from build123d import *

# Parameters (mm, degrees)
BOSS_EXTRUDE1_DEPTH = 8
SKETCH2_R           = 4.5
BOSS_EXTRUDE2_DEPTH = 7
CUT_EXTRUDE1_DEPTH  = 5.5
FILLET1_R           = 0.5
CHAMFER1_SIZE       = 0.25


with BuildPart() as part:
    # Sketch1 → Boss-Extrude1 (new body)
    with BuildSketch(Plane(origin=(0, 0, 0), x_dir=(1, 0, 0), z_dir=(0, 1, 0))):
        with BuildLine():
            Line((-1.75, 2.056088519), (-1.75, -2.056088519))
            ThreePointArc((-1.75, -2.056088519), (0, -2.7), (1.75, -2.056088519))
            Line((1.75, -2.056088519), (1.75, 2.056088519))
            ThreePointArc((1.75, 2.056088519), (0, 2.7), (-1.75, 2.056088519))
        make_face()
    extrude(amount=BOSS_EXTRUDE1_DEPTH)

    # Sketch2 → Boss-Extrude2 (add)
    with BuildSketch(Plane(origin=(0, 8, 0), x_dir=(1, 0, 0), z_dir=(0, 1, 0))):
        Circle(SKETCH2_R)
    extrude(amount=BOSS_EXTRUDE2_DEPTH)

    # Sketch3 → Cut-Extrude1 (cut)
    with BuildSketch(Plane(origin=(0, 15, 0), x_dir=(1, 0, 0), z_dir=(0, 1, 0))):
        with BuildLine():
            Line((-1.322875656, 1.5), (1.322875656, 1.5))
            ThreePointArc((1.322875656, 1.5), (0, -2), (-1.322875656, 1.5))
        make_face()
    extrude(amount=-CUT_EXTRUDE1_DEPTH, mode=Mode.SUBTRACT)

    # Fillet1
    fillet1_edges = [part.edges().sort_by_distance(p)[0] for p in [
        (0, 8, 2.7),
        (1.75, 8, 0),
        (0, 8, -2.7),
        (-1.75, 8, 0),
    ]]
    fillet(fillet1_edges, radius=FILLET1_R)

    # Chamfer1
    chamfer1_edges = [part.edges().sort_by_distance(p)[0] for p in [
        (-4.5, 8, 0),
        (-4.5, 15, 0),
        (0, 15, 2),
        (0, 15, -1.5),
        (1.75, 0, 0),
        (0, 0, 2.7),
        (-1.75, 0, 0),
        (0, 0, -2.7),
    ]]
    chamfer(chamfer1_edges, length=CHAMFER1_SIZE)


solid = part.part
Work out the finished part from the listing and answer in its coordinate system (mm). A direction names the side the tool comes from. Give positions to 0.01 mm unless a question says otherwise; leave off trailing zeros. Loops run counter-clockwise (first coordinate to the right, second up) from the corner with the lowest first, then second, coordinate; pieces in that order, holes last. Notation, with made-up numbers: (47, 56) -> (73, 56) arc R22 cw to (73, 64) -> close; hole circle Ø10 at (75.25, 89.5). An arc over 180 degrees is marked (long way). Use a Markdown table: item, result. Add a question column.
1. Section C-C on y = 5 is taken. Determine the outline of the cut face in (x, z), and give its area (3 significant figures).
2. Find the intervals of material crossed by probe 1 along X at (y, z) = (10.85, 0); probe 2 along Y at (x, z) = (0.25, 0); probe 3 along Y at (x, z) = (-3, 2), in increasing order.
3. Flat-ended cylindrical pins translate along their axes: pin 1 Ø4 at (x, y) = (-0.5, 11.5) entering from +Z; pin 2 Ø1.2 at (y, z) = (5.5, 0.5) entering from +X; pin 3 Ø1.2 at (y, z) = (3, -0.5) entering from -X; pin 4 Ø1.5 at (x, y) = (-1.5, 3.5) entering from +Z. Find the tip coordinate at first contact, or state that the pin passes through.
4. Section A-A on x = 0 is taken. Determine the outline of the cut face in (y, z), and give its area (3 significant figures).
5. Section B-B on z = 0 is taken. Determine the outline of the cut face in (x, y).
6. Determine the mould class of faces 1 (the cylindrical face through (0, 3.8, 2.7)), 2 (the flat face through (-1.75, 4, 0)), 3 (the cylindrical face through (0, 12, 2)) for opening direction Z: released by +Z, released by -Z, zero draft, split by the parting line, or undercut.
7. For faces 4 (the flat face through (3, 8, 0)), 5 (the flat face through (1.75, 4, 0)), 6 (the cylindrical face through (0, 3.8, -2.7)), 7 (the flat face through (0, 12, -1.5)), determine the directions among +Z, -Z, +X, -X, +Y, -Y from which every point of the face is accessible in a straight line to the end or side of a thin tool.
Results below:
| question | item | result |
|---|---|---|
| 1 | outline | (-1.75, -2.06) arc R2.7 ccw to (1.75, -2.06) -> (1.75, 2.06) arc R2.7 ccw to (-1.75, 2.06) -> close |
| 1 | area | 17.5 mm^2 |
| 2 | probe 1 | x = -4.5 to -2, 2 to 4.5 |
| 2 | probe 2 | y = 0 to 9.5 |
| 2 | probe 3 | y = 8 to 15 |
| 3 | pin 1 | stops at z = 4.5 |
| 3 | pin 2 | stops at x = 1.75 |
| 3 | pin 3 | stops at x = -1.75 |
| 3 | pin 4 | stops at z = 2.59 |
| 4 | outline | (0, -2.45) -> (0.25, -2.7) -> (7.5, -2.7) arc R0.5 cw to (8, -3.2) -> (8, -4.25) -> (8.25, -4.5) -> (14.75, -4.5) -> (15, -4.25) -> (15, -1.75) -> (14.75, -1.5) -> (9.5, -1.5) -> (9.5, 2) -> (14.75, 2) -> (15, 2.25) -> (15, 4.25) -> (14.75, 4.5) -> (8.25, 4.5) -> (8, 4.25) -> (8, 3.2) arc R0.5 cw to (7.5, 2.7) -> (0.25, 2.7) -> (0, 2.45) -> close |
| 4 | area | 86.8 mm^2 |
| 5 | outline | (-4.5, 8.25) -> (-4.25, 8) -> (-2.25, 8) arc R0.5 cw to (-1.75, 7.5) -> (-1.75, 0.25) -> (-1.5, 0) -> (1.5, 0) -> (1.75, 0.25) -> (1.75, 7.5) arc R0.5 cw to (2.25, 8) -> (4.25, 8) -> (4.5, 8.25) -> (4.5, 14.75) -> (4.25, 15) -> (2.25, 15) -> (2, 14.75) -> (2, 9.5) -> (-2, 9.5) -> (-2, 14.75) -> (-2.25, 15) -> (-4.25, 15) -> (-4.5, 14.75) -> close |
| 6 | face 1 | released by +Z |
| 6 | face 2 | zero draft |
| 6 | face 3 | undercut |
| 7 | face 4 | -Y |
| 7 | face 5 | +Z, -Z, +X, -Y |
| 7 | face 6 | -Z, -Y |
| 7 | face 7 | +Y |
